For this review, use the dimensioned drawing (mm, ordinates from the lowest corner) and the shaded views. A direction names the side the tool comes from. Round coordinates to 2 decimals unless told otherwise and drop trailing zeros. Write each loop counter-clockwise with the first axis right and the second up, starting at its lowest first coordinate (ties: lowest second). Pieces come first, ordered by that corner, then holes. Notation, with made-up numbers: M -10.5,-26.5 L -0.5,-26.5 A19 cw -0.5,-17.5 Z; hole C -9,28.5 d8. An arc over 180 degrees is marked long. One line per question, with ' | ' between items. Start each with the question number.
Item 1: Add section A-A, the plane y = 4. State the section outline as (x, z) points, and give its area (3 significant figures).
Item 2: For L1, parallel to X at y = 0.95, z = 2; L2, parallel to X at y = 4.45, z = 4.6; L3, parallel to Y at x = 19.5, z = 4.7, list the stretches that pass through material, from the lowest coordinate up.
Item 3: Add section C-C, the plane z = 4.8. State the section outline as (x, y) points.
Item 4: Insertion check: pin 1 Ø3 at (x, y) = (15.5, 4.5) entering from -Z. The pin has a flat end and moves straight along its axis. Give the tip position at first contact, or say it passes through.
Item 5: Add section D-D, the plane y = 0.75. State the section outline as (x, z) points, and give its area (3 significant figures).
Item 6: Add section B-B, the plane x = 19.5. State the section outline as (y, z) points.
Item 7: Machinability: for the marked faces 1 and 2, which of the approach directions +Z, -Z, +X, -X, +Y, -Y give a long, thin tool a straight path to every point of the face, cutting with its end or side? Answer none if there is none.
Item 8: Draft analysis for pull direction Y (two halves, no side actions). For the marked faces 3, 4, 5 and 6, state which applies: released by +Y, released by -Y, zero draft, split by the parting line, or undercut.
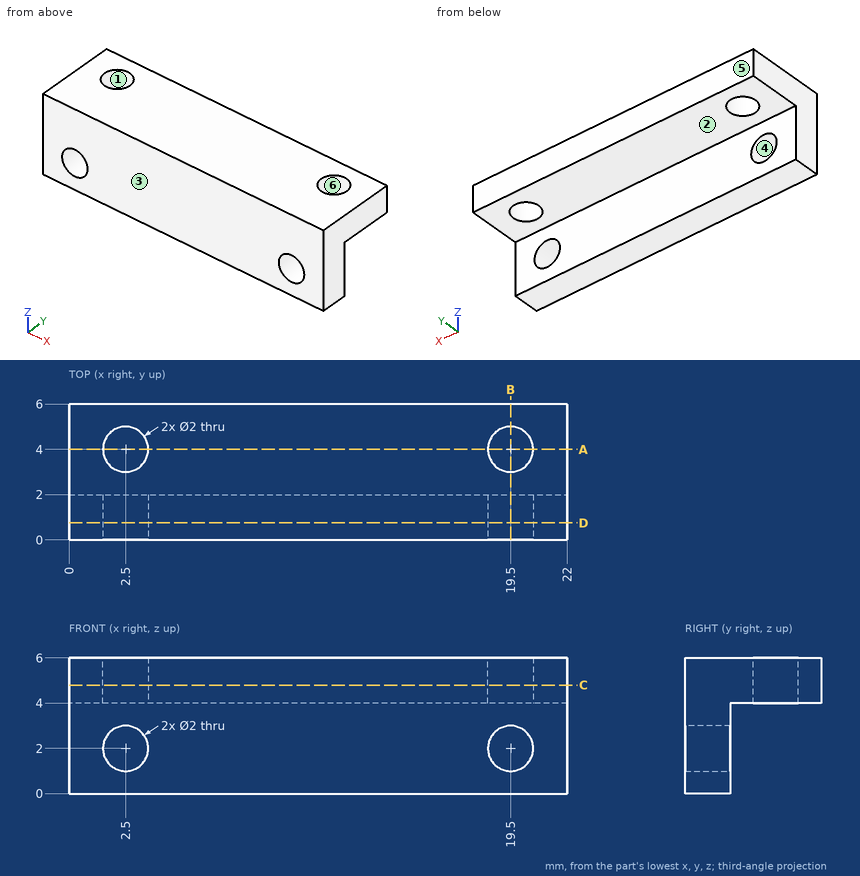
Computed values:
1) outline: M 0,4 L 1.5,4 L 1.5,6 L 0,6 Z; M 3.5,4 L 18.5,4 L 18.5,6 L 3.5,6 Z; M 20.5,4 L 22,4 L 22,6 L 20.5,6 Z | area: 36.0 mm^2
2) L1: x = 0 to 1.5, 3.5 to 18.5, 20.5 to 22 | L2: x = 0 to 1.61, 3.39 to 18.61, 20.39 to 22 | L3: y = 0 to 3, 5 to 6
3) outline: M 0,0 L 22,0 L 22,6 L 0,6 Z; hole C 2.5,4 d2; hole C 19.5,4 d2
4) pin 1: stops at z = 4
5) outline: M 0,0 L 22,0 L 22,6 L 0,6 Z; hole C 2.5,2 d2; hole C 19.5,2 d2 | area: 126 mm^2
6) outline: M 0,0 L 2,0 L 2,1 L 0,1 Z; M 0,3 L 2,3 L 2,4 L 3,4 L 3,6 L 0,6 Z; M 5,4 L 6,4 L 6,6 L 5,6 Z
7) face 1: +Z, -Z | face 2: -Z, +X, -X, +Y
8) face 3: released by -Y | face 4: zero draft | face 5: released by +Y | face 6: undercut
